For this review, use the dimensioned drawing (mm, ordinates from the lowest corner) and the shaded views. A direction names the side the tool comes from. Round coordinates to 2 decimals unless told otherwise and drop trailing zeros. Write each loop counter-clockwise with the first axis right and the second up, starting at its lowest first coordinate (ties: lowest second). Pieces come first, ordered by that corner, then holes. Notation, with made-up numbers: (46.5, 61) -> (83.5, 61) arc R19 ccw to (83.5, 77) -> close; hole circle Ø11 at (-37.5, 66.25). An arc over 180 degrees is marked (long way). Answer in a Markdown table with one row per item. Add a question column.
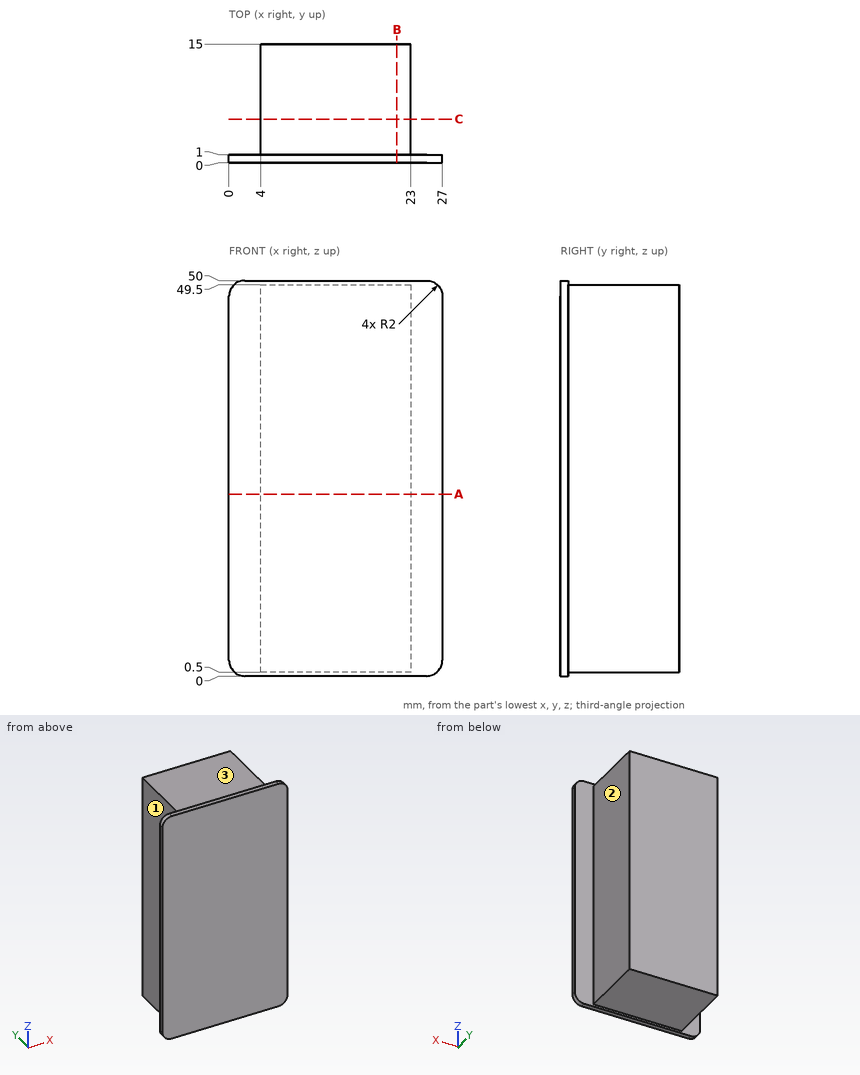
1. We need section B-B (x = 21.25). Write out the cut boundary in (y, z), plus the area to 3 significant figures.
2. Tool access review of the marked faces 1, 2 and 3: name each direction out of +Z, -Z, +X, -X, +Y, -Y from which nothing blocks a thin tool from reaching the whole face with its end or side.
3. Clearance check with flat-ended pins moving along their axes: pin 1 Ø2 at (x, y) = (4, 11) entering from +Z; pin 2 Ø2 at (y, z) = (9, 25.5) entering from -X; pin 3 Ø8 at (x, y) = (15, 5.5) entering from -Z. State where each tip first meets the part, or that it passes through.
4. We need section A-A (z = 23). Write out the cut boundary in (x, y).
5. We need section C-C (y = 5.5). Write out the cut boundary in (x, z), plus the area to 3 significant figures.
6. For L1, parallel to Z at x = 16.5, y = 10.25; L2, parallel to X at y = 7, z = 25; L3, parallel to Y at x = 1.75, z = 36, list the stretches that pass through material, from the lowest coordinate up. Write a range as [from, to].
Response:
| question | item | result |
|---|---|---|
| 1 | outline | (0, 0) -> (1, 0) -> (1, 0.5) -> (15, 0.5) -> (15, 49.5) -> (1, 49.5) -> (1, 50) -> (0, 50) -> close |
| 1 | area | 736 mm2 |
| 2 | face 1 | +Z, -Z, -X, +Y |
| 2 | face 2 | +Z, -Z, +X, +Y |
| 2 | face 3 | +Z, +X, -X, +Y |
| 3 | pin 1 | z = 49.5 |
| 3 | pin 2 | x = 4 |
| 3 | pin 3 | z = 0.5 |
| 4 | outline | (0, 0) -> (27, 0) -> (27, 1) -> (23, 1) -> (23, 15) -> (4, 15) -> (4, 1) -> (0, 1) -> close |
| 5 | outline | (4, 0.5) -> (23, 0.5) -> (23, 49.5) -> (4, 49.5) -> close |
| 5 | area | 931 mm2 |
| 6 | L1 | [0.5, 49.5] |
| 6 | L2 | [4, 23] |
| 6 | L3 | [0, 1] |
